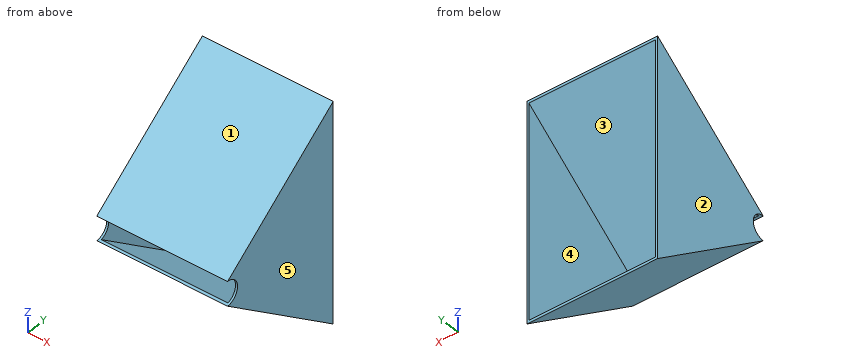
from build123d import *

# Parameters (mm, degrees)
BOSS_EXTRUDE1_DEPTH = 101.6
SHELL3_T            = -1.5875


with BuildPart() as part:
    # Sketch1 → Boss-Extrude1 (new body)
    with BuildSketch(Plane(origin=(0, 0, 0), x_dir=(0, 0, -1), z_dir=(1, 0, 0))):
        with BuildLine():
            Line((-9.525, 0), (-85.725, 101.6))
            Line((-85.725, 101.6), (85.725, 101.6))
            Line((85.725, 101.6), (9.525, 0))
            ThreePointArc((9.525, 0), (0, 9.525), (-9.525, 0))
        make_face()
    extrude(amount=BOSS_EXTRUDE1_DEPTH)

    # Shell3
    shell3_openings = [part.faces().sort_by_distance(p)[0] for p in [
        (50.8, 101.6, 0),
        (50.8, 4.7625, 0),
    ]]
    offset(amount=SHELL3_T, openings=shell3_openings, kind=Kind.INTERSECTION)


solid = part.part
The listing builds one solid part. Answer for the finished solid, in the listing's coordinates (mm). Face numbers are marked on the shaded views. A direction names the side the tool comes from. Round coordinates to 2 decimals unless told otherwise and drop trailing zeros. Loops run counter-clockwise (first coordinate to the right, second up) from the corner with the lowest first, then second, coordinate; pieces in that order, holes last. Notation, with made-up numbers: M 69.25,11 L 89.25,11 A12 cw 89.25,28 Z; hole C 82,1.5 d3. An arc over 180 degrees is marked long. Return JSON: item names as keys, results as strings.
Q1. Find section B-B, the plane x = 59. Determine the outline of the cut face in (y, z) (3 decimals).
Results list:
{"outline": "M 0,-9.525 L 101.6,-85.725 L 101.6,-83.741 L 2.277,-9.249 A9.525 cw Z; M 0,9.525 A9.525 cw 2.277,9.249 L 101.6,83.741 L 101.6,85.725 Z"}
Q2. Find section C-C, the plane y = 81. Determine the outline of the cut face in (x, z) (1 decimal), plus the area to 3 significant figures.
Results list:
{"outline": "M 0,-70.3 L 101.6,-70.3 L 101.6,70.3 L 0,70.3 Z; hole M 1.6,-68.3 L 100,-68.3 L 100,68.3 L 1.6,68.3 Z", "area": "837 mm2"}
Q3. Find the intervals of material crossed by line 1 along X through (y, z) = (67.5, -3); line 2 along Z through (x, y) = (77, 87) (3 decimals); line 3 along Z through (x, y) = (98, 38.5), in increasing order. Write a range as from..to.
Results list:
{"line 1": "x = 0..1.59, 100.01..101.6", "line 2": "z = -74.775..-72.791, 72.791..74.775", "line 3": "z = -38.4..-36.42, 36.42..38.4"}
Q4. Each of these flat-tipped pins is pushed along its axis until it touches: pin 1 Ø1 at (x, y) = (12, 43.5) entering from +Z (3 decimals); pin 2 Ø10 at (x, z) = (86.5, 14) entering from -Y; pin 3 Ø6 at (x, z) = (78.5, 6.5) entering from +Y. Where does it stop, or does it pass through?
Results list:
{"pin 1": "stops at z = 42.525", "pin 2": "stops at y = 0", "pin 3": "stops at y = 2.61"}
Q5. Find section A-A, the plane z = 0. Determine the outline of the cut face in (x, y) (1 decimal), plus the area to 3 significant figures.
Results list:
{"outline": "M 0,9.5 L 1.6,9.5 L 1.6,101.6 L 0,101.6 Z; M 100,9.5 L 101.6,9.5 L 101.6,101.6 L 100,101.6 Z", "area": "292 mm2"}
Q6. Which of the six approach directions +Z, -Z, +X, -X, +Y, -Y give full straight-line access (tool end or side, diameter ignored) to the marked faces 4 and 5?
Results list:
{"face 4": "+Y", "face 5": "+Z, -Z, +X, +Y, -Y"}
Q7. Find section D-D, the plane z = -48. Determine the outline of the cut face in (x, y), plus the area to 3 significant figures.
Results list:
{"outline": "M 0,51.3 L 101.6,51.3 L 101.6,101.6 L 100.01,101.6 L 100.01,53.95 L 1.59,53.95 L 1.59,101.6 L 0,101.6 Z", "area": "420 mm2"}
Q8. The mould has two halves that part along Z. Classify the marked faces 1, 2 and 3: released by +Z, released by -Z, zero draft, split by the parting line, or undercut.
Results list:
{"face 1": "released by +Z", "face 2": "zero draft", "face 3": "undercut"}
